from build123d import *

# Parameters (mm, degrees)
SKETCH1_R               = 32.5
BOSS_EXTRUDE1_DEPTH     = 3
CUT_EXTRUDE1_DEPTH      = 10
CUT_EXTRUDE1_DEPTH_BACK = 47.059743812
SKETCH2_R               = 3.5
SKETCH2_W               = 6.5
SKETCH2_H               = 6.5


with BuildPart() as part:
    # Sketch1 → Boss-Extrude1 (new body)
    with BuildSketch(Plane(origin=(0, 0, 0), x_dir=(1, 0, 0), z_dir=(0, 1, 0))):
        with Locations(Location((0, 0, 0), (0, 0, 270))):
            Circle(SKETCH1_R)
    extrude(amount=BOSS_EXTRUDE1_DEPTH)

    # Sketch2 → Cut-Extrude1 (cut, two sides: drawn at the far end of the back side and taken through both)
    with BuildSketch(Plane(origin=(0, 0, 0), x_dir=(1, 0, 0), z_dir=(0, 1, 0)).offset(-CUT_EXTRUDE1_DEPTH_BACK)):
        with Locations(Location((0, 0, 0), (0, 0, 270))):
            Circle(SKETCH2_R)
        with Locations((0, -27.5)):
            Rectangle(SKETCH2_W, SKETCH2_H)
        with Locations((27.5, 0)):
            Rectangle(SKETCH2_W, SKETCH2_H)
        with Locations((-27.5, 0)):
            Rectangle(SKETCH2_W, SKETCH2_H)
        with Locations((0, 27.5)):
            Rectangle(SKETCH2_W, SKETCH2_H)
    extrude(amount=CUT_EXTRUDE1_DEPTH + CUT_EXTRUDE1_DEPTH_BACK, mode=Mode.SUBTRACT)


solid = part.part
Could you check a few things on this model? Use its own coordinates, in mm. Round coordinates to 2 decimals unless told otherwise and drop trailing zeros. Order: outer loops, then holes, each group sorted by start corner. A loop starts at its lowest first (then second) coordinate and runs counter-clockwise, first axis right, second up.
Q1. Thinking about a two-plate mould opening in Z: for faces 1 (the face through (0, 0, 7)), 2 (the face through (-3.417, 1.479, -0.759)), which applies, released by +Z, released by -Z, zero draft, split by the parting line, or undercut?
Geometry says:
face 1: zero draft
face 2: undercut
Q2. Imagine slicing it at B-B, the plane x = -28. List the corners of the cut face in (y, z) for me, then the cut area to 3 significant figures.
Geometry says:
outline: (0, -16.5) - (3, -16.5) - (3, -3.25) - (0, -3.25) - close; (0, 3.25) - (3, 3.25) - (3, 16.5) - (0, 16.5) - close
area: 79.5 mm2
Q3. Imagine slicing it at D-D, the plane y = 0.95. List the corners of the cut face in (x, z) for me, then the cut area to 3 significant figures.
Geometry says:
outline: circle Ø65 at (0, 0); hole (-30.75, -3.25) - (-24.25, -3.25) - (-24.25, 3.25) - (-30.75, 3.25) - close; hole circle Ø7 at (0, 0); hole (-3.25, -30.75) - (3.25, -30.75) - (3.25, -24.25) - (-3.25, -24.25) - close; hole (-3.25, 24.25) - (3.25, 24.25) - (3.25, 30.75) - (-3.25, 30.75) - close; hole (24.25, -3.25) - (30.75, -3.25) - (30.75, 3.25) - (24.25, 3.25) - close
area: 3,110 mm2
Q4. Please list where these lines run through material, in increasing order: probe 1 along X at (y, z) = (2.35, 0); probe 2 along Z at (x, y) = (-1, 0.95); probe 3 along Z at (x, y) = (-3, 1.9).
Geometry says:
probe 1: x = -32.5 to -30.75, -24.25 to -3.5, 3.5 to 24.25, 30.75 to 32.5
probe 2: z = -32.48 to -30.75, -24.25 to -3.35, 3.35 to 24.25, 30.75 to 32.48
probe 3: z = -32.36 to -30.75, -24.25 to -1.8, 1.8 to 24.25, 30.75 to 32.36
Q5. Imagine slicing it at A-A, the plane z = 0. List the corners of the cut face in (x, y) for me, then the cut area to 3 significant figures.
Geometry says:
outline: (-32.5, 0) - (-30.75, 0) - (-30.75, 3) - (-32.5, 3) - close; (-24.25, 0) - (-3.5, 0) - (-3.5, 3) - (-24.25, 3) - close; (3.5, 0) - (24.25, 0) - (24.25, 3) - (3.5, 3) - close; (30.75, 0) - (32.5, 0) - (32.5, 3) - (30.75, 3) - close
area: 135 mm2
Q6. I'm going to push flat-ended pins straight in: P1, Ø1.5, axis at y = 1, z = -27.5, coming from the +X side; P2, Ø0.9, axis at x = -0.5, y = 2, coming from the -Z side; P3, Ø1.5, axis at x = -26, y = 1.5, coming from the +Z side; P4, Ø1, axis at y = 1, z = -15.5, coming from the +X side. Where does each tip first touch, or does it pass through?
Geometry says:
P1: stops at x = 18.46
P2: stops at z = -32.5
P3: stops at z = 20.46
P4: stops at x = 28.83
Q7. Imagine slicing it at C-C, the plane x = 0. List the corners of the cut face in (y, z) for me, then the cut area to 3 significant figures.
Geometry says:
outline: (0, -32.5) - (3, -32.5) - (3, -30.75) - (0, -30.75) - close; (0, -24.25) - (3, -24.25) - (3, -3.5) - (0, -3.5) - close; (0, 3.5) - (3, 3.5) - (3, 24.25) - (0, 24.25) - close; (0, 30.75) - (3, 30.75) - (3, 32.5) - (0, 32.5) - close
area: 135 mm2
